```python
from build123d import *

# Parameters (mm, degrees)
F1_DEPTH = 63.5
F3_DEPTH = 57.15
F4_DEPTH = 127
F5_DEPTH = 101.6


with BuildPart() as f1:
    # F0 (on Front) → F1 (new body, symmetric)
    with BuildSketch(Plane.XZ):
        Polygon((127, 0), (63.5, 109.985226), (-63.5, 109.985226), (-127, 0), (-63.5, -109.985226), (63.5, -109.985226), align=None)
        Polygon((-66.799852, -84.545206), (-66.799852, 85.417562), (-18.633867, 85.417562), (-18.633867, 9.979562), (11.241462, 84.802525), (64.756104, 84.802525), (30.896133, 0), (64.756104, -84.802525), (11.241462, -84.802525), (-18.633867, -9.979562), (-18.633867, -84.545206), align=None, mode=Mode.SUBTRACT)
    extrude(amount=F1_DEPTH, both=True)

    # F2 (on Top) → F3 (cut)
    with BuildSketch(Plane.XY):
        Polygon((-81.175185, 15.08125), (-83.924815, 15.08125), (-85.299631, 12.7), (-83.924815, 10.31875), (-81.175185, 10.31875), (-79.800369, 12.7), align=None)
        Polygon((-81.250962, -10.45), (-83.849038, -10.45), (-85.148076, -12.7), (-83.849038, -14.95), (-81.250962, -14.95), (-79.951924, -12.7), align=None)
        Polygon((-81.404321, -36.115625), (-83.695679, -36.115625), (-84.841359, -38.1), (-83.695679, -40.084375), (-81.404321, -40.084375), (-80.258641, -38.1), align=None)
        Polygon((-85.436751, 37.998921), (-83.905839, 35.549461), (-81.019088, 35.650539), (-79.663249, 38.201079), (-81.194161, 40.650539), (-84.080912, 40.549461), align=None)
        Polygon((79.663249, 38.201079), (81.019088, 35.650539), (83.905839, 35.549461), (85.436751, 37.998921), (84.080912, 40.549461), (81.194161, 40.650539), align=None)
        Polygon((83.924815, 10.31875), (85.299631, 12.7), (83.924815, 15.08125), (81.175185, 15.08125), (79.800369, 12.7), (81.175185, 10.31875), align=None)
        Polygon((81.250962, -10.45), (79.951924, -12.7), (81.250962, -14.95), (83.849038, -14.95), (85.148076, -12.7), (83.849038, -10.45), align=None)
        Polygon((81.404321, -40.084375), (83.695679, -40.084375), (84.841359, -38.1), (83.695679, -36.115625), (81.404321, -36.115625), (80.258641, -38.1), align=None)
    extrude(amount=-F3_DEPTH, mode=Mode.SUBTRACT)

    # F2 (on Top) → F4 (cut)
    with BuildSketch(Plane.XY):
        Polygon((-85.436751, 37.998921), (-83.905839, 35.549461), (-81.019088, 35.650539), (-79.663249, 38.201079), (-81.194161, 40.650539), (-84.080912, 40.549461), align=None)
        Polygon((-81.175185, 15.08125), (-83.924815, 15.08125), (-85.299631, 12.7), (-83.924815, 10.31875), (-81.175185, 10.31875), (-79.800369, 12.7), align=None)
        Polygon((-81.250962, -10.45), (-83.849038, -10.45), (-85.148076, -12.7), (-83.849038, -14.95), (-81.250962, -14.95), (-79.951924, -12.7), align=None)
        Polygon((-81.404321, -36.115625), (-83.695679, -36.115625), (-84.841359, -38.1), (-83.695679, -40.084375), (-81.404321, -40.084375), (-80.258641, -38.1), align=None)
        Polygon((81.250962, -10.45), (79.951924, -12.7), (81.250962, -14.95), (83.849038, -14.95), (85.148076, -12.7), (83.849038, -10.45), align=None)
        Polygon((81.404321, -40.084375), (83.695679, -40.084375), (84.841359, -38.1), (83.695679, -36.115625), (81.404321, -36.115625), (80.258641, -38.1), align=None)
        Polygon((83.924815, 10.31875), (85.299631, 12.7), (83.924815, 15.08125), (81.175185, 15.08125), (79.800369, 12.7), (81.175185, 10.31875), align=None)
        Polygon((79.663249, 38.201079), (81.019088, 35.650539), (83.905839, 35.549461), (85.436751, 37.998921), (84.080912, 40.549461), (81.194161, 40.650539), align=None)
        Polygon((0.12826, 41.979922), (5.062896, 44.977038), (4.934636, 50.749116), (-0.12826, 53.524078), (-5.062896, 50.526962), (-4.934636, 44.754884), align=None)
        Polygon((-0.000787, 23.18495), (4.762107, 25.933899), (4.762893, 31.43316), (0.000787, 34.183472), (-4.762107, 31.434523), (-4.762893, 25.935262), align=None)
        Polygon((4, 7.29941), (4, 11.918212), (0, 14.227613), (-4, 11.918212), (-4, 7.29941), (0, 4.990009), align=None)
        Polygon((-0.000656, -14.049307), (3.968422, -11.758516), (3.969078, -7.175798), (0.000656, -4.883871), (-3.968422, -7.174662), (-3.969078, -11.75738), align=None)
        Polygon((3.175, -30.375076), (3.175, -26.708902), (0, -24.875815), (-3.175, -26.708902), (-3.175, -30.375076), (0, -32.208163), align=None)
        Polygon((3, -49.34944), (3, -45.885338), (0, -44.153287), (-3, -45.885338), (-3, -49.34944), (0, -51.081491), align=None)
    extrude(amount=F4_DEPTH, mode=Mode.SUBTRACT)

    # F2 (on Top) → F5 (cut)
    with BuildSketch(Plane.XY):
        Polygon((-0.000656, -14.049307), (3.968422, -11.758516), (3.969078, -7.175798), (0.000656, -4.883871), (-3.968422, -7.174662), (-3.969078, -11.75738), align=None)
        Polygon((3.175, -30.375076), (3.175, -26.708902), (0, -24.875815), (-3.175, -26.708902), (-3.175, -30.375076), (0, -32.208163), align=None)
        Polygon((4, 7.29941), (4, 11.918212), (0, 14.227613), (-4, 11.918212), (-4, 7.29941), (0, 4.990009), align=None)
        Polygon((-0.000787, 23.18495), (4.762107, 25.933899), (4.762893, 31.43316), (0.000787, 34.183472), (-4.762107, 31.434523), (-4.762893, 25.935262), align=None)
        Polygon((3, -49.34944), (3, -45.885338), (0, -44.153287), (-3, -45.885338), (-3, -49.34944), (0, -51.081491), align=None)
        Polygon((0.12826, 41.979922), (5.062896, 44.977038), (4.934636, 50.749116), (-0.12826, 53.524078), (-5.062896, 50.526962), (-4.934636, 44.754884), align=None)
    extrude(amount=-F5_DEPTH, mode=Mode.SUBTRACT)


solid = f1.part
```
Geometry: final body of the model. Coordinates: model frame, mm. A direction names the side the tool comes from. Give positions to 0.01 mm unless a question says otherwise; leave off trailing zeros. Order: outer loops, then holes, each group sorted by start corner. A loop starts at its lowest first (then second) coordinate and runs counter-clockwise, first axis right, second up. Notation, with made-up numbers: (33.25, 84) -> (72.25, 84) arc R10 cw to (72.25, 89) -> close; hole circle Ø10 at (88, 50). An arc over 180 degrees is marked (long way). Write each question's results on one line, items separated by ' | '. Start each with the question number.
1) Draft query along X for faces 4 (the flat face through (94.806, -0.889, -55.763)), 5 (the flat face through (0, -9, -101.6)), 6 (the flat face through (-94.806, -0.889, 55.763)). Return one class per face: pulls with the +X half, pulls with the -X half, needs draft (parallel to the pull), parting line crosses it, or undercut.
2) First-contact query: pin 1 (5 mm diameter, centred on x = -81.5, y = -12, fed in from +Z); pin 2 (2.5 mm diameter, centred on y = -9, z = -78.5, fed in from -X); pin 3 (2.5 mm diameter, centred on y = 10.5, z = -73, fed in from +X). Flat tips, straight axial feed; report the tip coordinate or a pass-through.
3) Section A-A (y = -54). Return loops of the section in (x, z), then the cut area to 3 significant figures.
4) Section C-C (x = 41.5). Return loops of the section in (y, z), then the cut area to 3 significant figures.
5) Line query: line 1 (Y direction, x = 80.5, z = -16); line 2 (X direction, y = -38.5, z = -43.5); line 3 (X direction, y = 3, z = -23). Output: solid intervals per line, ascending. Write a range as from..to.
6) Section B-B (x = -48). Return loops of the section in (y, z), then the cut area to 3 significant figures.
7) Section D-D (z = -26). Count the separate pieces of the cut face and the enclosed holes in it, then the cut area to 3 significant figures.
8) Set-up query: faces 1 (the flat face through (0, 48, -101.6)), 2 (the flat face through (95.694, -0.889, 54.223)), 3 (the flat face through (38, -1, -84.803)). Return all of +Z, -Z, +X, -X, +Y, -Y with unobstructed straight access to the full face (end or side cutting, diameter ignored); none if empty.
Calculated:
1) face 4: pulls with the +X half | face 5: undercut | face 6: pulls with the -X half
2) pin 1: z = 83.14 | pin 2: x = -82.4 | pin 3: x = 85.58
3) outline: (-127, 0) -> (-63.5, -109.99) -> (63.5, -109.99) -> (127, 0) -> (63.5, 109.99) -> (-63.5, 109.99) -> close; hole (-66.8, -84.55) -> (-18.63, -84.55) -> (-18.63, -9.98) -> (11.24, -84.8) -> (64.76, -84.8) -> (30.9, 0) -> (64.76, 84.8) -> (11.24, 84.8) -> (-18.63, 9.98) -> (-18.63, 85.42) -> (-66.8, 85.42) -> close | area: 24,700 mm2
4) outline: (-63.5, -109.99) -> (63.5, -109.99) -> (63.5, -84.8) -> (-63.5, -84.8) -> close; (-63.5, -26.56) -> (63.5, -26.56) -> (63.5, 26.56) -> (-63.5, 26.56) -> close; (-63.5, 84.8) -> (63.5, 84.8) -> (63.5, 109.99) -> (-63.5, 109.99) -> close | area: 13,100 mm2
5) line 1: -63.5..-38.52, -37.68..-13.65, -11.75..11.49, 13.91..36.63, 39.54..63.5 | line 2: -101.89..-84.61, -80.49..-66.8, -18.63..-5.25, 48.26..80.49, 84.61..101.89 | line 3: -113.72..-66.8, -18.63..-13.44, 40.08..113.72
6) outline: (-63.5, -109.99) -> (63.5, -109.99) -> (63.5, -84.55) -> (-63.5, -84.55) -> close; (-63.5, 85.42) -> (63.5, 85.42) -> (63.5, 109.99) -> (-63.5, 109.99) -> close | area: 6,350 mm2
7) separate pieces: 3 | enclosed holes: 8 | area: 15,400 mm2
8) face 1: +Z | face 2: +Z, +X, +Y, -Y | face 3: +Y, -Y
